Build history of the part. All positions in model axes, mm. A direction names the side the tool comes from. Give positions to 0.01 mm unless a question says otherwise; leave off trailing zeros. Order: outer loops, then holes, each group sorted by start corner. A loop starts at its lowest first (then second) coordinate and runs counter-clockwise, first axis right, second up. Notation, with made-up numbers: M 33,70 L 82,70 A30 ccw 82,98 Z; hole C 37,39.5 d1. An arc over 180 degrees is marked long. One line per item, written item: value.
from build123d import *

# Parameters (mm, degrees)
SKETCH2_R                = 37.75
SKETCH2_R_2              = 7.75
BOSS_EXTRUDE1_DEPTH      = 30
SKETCH3_R                = 1
CUT_EXTRUDE1_DEPTH       = 10
SKETCH4_R                = 1.5
BOSS_EXTRUDE2_DEPTH      = 5
FILLET1_R                = 10
CIRPATTERN1_COUNT        = 4
FILLET1_OF_CIRPATTERN1_R = 10


with BuildPart() as part:
    # Sketch2 → Boss-Extrude1 (new body)
    with BuildSketch(Plane.XY):
        Circle(SKETCH2_R)
        Circle(SKETCH2_R_2, mode=Mode.SUBTRACT)
    extrude(amount=BOSS_EXTRUDE1_DEPTH)

    # Sketch3 → Cut-Extrude1 (cut)
    with BuildSketch(Plane.XY.offset(30)):
        with Locations((0, 12.5)):
            Circle(SKETCH3_R)
        with Locations((10.825317547, -6.25)):
            Circle(SKETCH3_R)
        with Locations((-10.825317547, -6.25)):
            Circle(SKETCH3_R)
    extrude(amount=-CUT_EXTRUDE1_DEPTH, mode=Mode.SUBTRACT)

    # Sketch4 → Boss-Extrude2 (add)
    with BuildSketch(Plane(origin=(0, 0, 0), x_dir=(-1, 0, 0), z_dir=(0, 0, -1))):
        with BuildLine():
            Line((-4, 37.495028442), (0, 37.75))
            Line((0, 37.75), (4, 37.495028442))
            Line((4, 37.495028442), (4, 40))
            ThreePointArc((4, 40), (0, 44), (-4, 40))
            Line((-4, 40), (-4, 37.495028442))
        make_face()
        with Locations((0, 40)):
            Circle(SKETCH4_R, mode=Mode.SUBTRACT)
    boss_extrude2 = extrude(amount=-BOSS_EXTRUDE2_DEPTH)

    # Fillet1
    # the kernel refuses this fillet: 10 mm, written as the material it adds along each edge
    with BuildSketch(Plane(origin=(4, 37.537481269, 5), x_dir=(0.9825908408243521, -0.18578277511139904, 0), z_dir=(0, 0, -1))) as fillet1_piece_1:
        with BuildLine():
            CenterArc((6.893121156, -9.967448048), FILLET1_R, 94.624278966, 49.061773925)
            Line((-1.164720332, -4.045354621), (-1.970504481, -3.453145278))
            ThreePointArc((-1.970504481, -3.453145278), (-1.440084404, -2.233865576), (-0.982590841, 0.185782775))
            Line((-0.982590841, 0.185782775), (0.0806213, 0.996744805))
            ThreePointArc((0.0806213, 0.996744805), (3.043454077, 0.877116383), (6.006286855, 0.996744805))
            Line((6.006286855, 0.996744805), (6.086908155, 0))
        make_face()
    extrude(amount=5)
    with BuildSketch(Plane(origin=(-4, 37.537481269, 5), x_dir=(-0.9825908408243521, -0.185782775111399, 0), z_dir=(0, 0, -1))) as fillet1_piece_2:
        with BuildLine():
            CenterArc((6.893121156, 9.967448048), FILLET1_R, 216.31394711, 49.061773925)
            Line((-1.164720332, 4.045354621), (-1.970504481, 3.453145278))
            ThreePointArc((-1.970504481, 3.453145278), (-1.440084404, 2.233865576), (-0.982590841, -0.185782775))
            Line((-0.982590841, -0.185782775), (0.0806213, -0.996744805))
            ThreePointArc((0.0806213, -0.996744805), (3.043454077, -0.877116383), (6.006286855, -0.996744805))
            Line((6.006286855, -0.996744805), (6.086908155, 0))
        make_face()
    extrude(amount=5)

    # CirPattern1: Boss-Extrude2 ×4 about axis
    cirpattern1_axis = Axis((0, 0, 0), (0, 0, 1))
    for i in range(1, CIRPATTERN1_COUNT):
        add(boss_extrude2.rotate(cirpattern1_axis, i * 360 / CIRPATTERN1_COUNT))

    # Fillet1 of CirPattern1
    # the kernel refuses this fillet: 10 mm, written as the material it adds along each edge
    with BuildSketch(Plane(origin=(-37.537481269, 4, 5), x_dir=(0.18578277511140276, 0.9825908408243514, 0), z_dir=(0, 0, -1)), Plane(origin=(-4, -37.537481269, 5), x_dir=(-0.9825908408243512, 0.18578277511140392, 0), z_dir=(0, 0, -1)), Plane(origin=(37.537481269, -4, 5), x_dir=(-0.1857827751114012, -0.9825908408243518, 0), z_dir=(0, 0, -1))) as fillet1_of_cirpattern1_piece_1:
        with BuildLine():
            CenterArc((6.893121156, -9.967448048), FILLET1_OF_CIRPATTERN1_R, 94.624278966, 49.061773925)
            Line((-1.164720332, -4.045354621), (-1.970504481, -3.453145278))
            ThreePointArc((-1.970504481, -3.453145278), (-1.440084404, -2.233865576), (-0.982590841, 0.185782775))
            Line((-0.982590841, 0.185782775), (0.0806213, 0.996744805))
            ThreePointArc((0.0806213, 0.996744805), (3.043454077, 0.877116383), (6.006286855, 0.996744805))
            Line((6.006286855, 0.996744805), (6.086908155, 0))
        make_face()
    extrude(amount=5)
    with BuildSketch(Plane(origin=(-37.537481269, -4, 5), x_dir=(0.1857827751113977, -0.9825908408243523, 0), z_dir=(0, 0, -1)), Plane(origin=(4, -37.537481269, 5), x_dir=(0.9825908408243529, 0.18578277511139504, 0), z_dir=(0, 0, -1)), Plane(origin=(37.537481269, 4, 5), x_dir=(-0.18578277511139632, 0.9825908408243527, 0), z_dir=(0, 0, -1))) as fillet1_of_cirpattern1_piece_2:
        with BuildLine():
            CenterArc((6.893121156, 9.967448048), FILLET1_OF_CIRPATTERN1_R, 216.31394711, 49.061773925)
            Line((-1.164720332, 4.045354621), (-1.970504481, 3.453145278))
            ThreePointArc((-1.970504481, 3.453145278), (-1.440084404, 2.233865576), (-0.982590841, -0.185782775))
            Line((-0.982590841, -0.185782775), (0.0806213, -0.996744805))
            ThreePointArc((0.0806213, -0.996744805), (3.043454077, -0.877116383), (6.006286855, -0.996744805))
            Line((6.006286855, -0.996744805), (6.086908155, 0))
        make_face()
    extrude(amount=5)


solid = part.part
1) Saw through at A-A, the plane z = 3.5. Write the cut outline in (x, y), then the cut area to 3 significant figures.
Check values:
outline: M -41.73,-3.61 A10 cw -36.41,-9.98 A37.75 ccw -9.98,-36.41 A10 cw -3.61,-41.73 A4 ccw 3.61,-41.73 A10 cw 9.98,-36.41 A37.75 ccw 36.41,-9.98 A10 cw 41.73,-3.61 A4 ccw 41.73,3.61 A10 cw 36.41,9.98 A37.75 ccw 9.98,36.41 A10 cw 3.61,41.73 A4 ccw -3.61,41.73 A10 cw -9.98,36.41 A37.75 ccw -36.41,9.98 A10 cw -41.73,3.61 A4 ccw Z; hole C -40,0 d3; hole C 0,0 d15.5; hole C 0,-40 d3; hole C 0,40 d3; hole C 40,0 d3
area: 4,480 mm^2
2) Saw through at B-B, the plane y = 0. Write the cut outline in (x, z).
Check values:
outline: M -44,0 L -41.5,0 L -41.5,5 L -44,5 Z; M -38.5,0 L -7.75,0 L -7.75,30 L -37.75,30 L -37.75,5 L -38.5,5 Z; M 7.75,0 L 38.5,0 L 38.5,5 L 37.75,5 L 37.75,30 L 7.75,30 Z; M 41.5,0 L 44,0 L 44,5 L 41.5,5 Z
3) Drill centre lines: probe 1 along Y at (x, z) = (0, 3.05); probe 2 along Y at (x, z) = (10, 26.5); probe 3 along Y at (x, z) = (0, 19). Where is each one in solid material? Low to high. Write a range as from..to.
Check values:
probe 1: -44..-41.5, -38.5..-7.75, 7.75..38.5, 41.5..44
probe 2: -36.4..-6.81, -5.69..36.4
probe 3: -37.75..-7.75, 7.75..37.75
4) Saw through at D-D, the plane z = 24. Write the cut outline in (x, y), then the cut area to 3 significant figures.
Check values:
outline: C 0,0 d75.5; hole C -10.83,-6.25 d2; hole C 0,0 d15.5; hole C 0,12.5 d2; hole C 10.83,-6.25 d2
area: 4,280 mm^2
5) Tool access for faces 1 (the face through (6.17, -38.413, 2.535)), 2 (the face through (11, -6, 20)): list every direction of +Z, -Z, +X, -X, +Y, -Y with a clear straight run to the whole face (end or side of a thin tool).
Check values:
face 1: +Z, -Z, +X, -Y
face 2: +Z
6) Saw through at C-C, the plane x = 5. Write the cut outline in (y, z), then the cut area to 3 significant figures.
Check values:
outline: M -39.58,0 L -5.92,0 L -5.92,30 L -37.42,30 L -37.42,5 L -39.58,5 Z; M 5.92,0 L 39.58,0 L 39.58,5 L 37.42,5 L 37.42,30 L 5.92,30 Z
area: 1,910 mm^2
7) Pin check, flat tips, straight feed: pin 1 (4 mm diameter, centred on x = -40, y = -3.5, fed in from +Z); pin 2 (2 mm diameter, centred on y = -30, z = 18, fed in from +X); pin 3 (5 mm diameter, centred on x = 11, z = 9, fed in from -Y). Stop position of each tip, or through.
Check values:
pin 1: z = 5
pin 2: x = 24.17
pin 3: y = -36.78
8) Mould opens along Y. For faces 3 (the face through (0, -44, 2)), 4 (the face through (-1.009, 7.684, 14.79)), 5 (the face through (36.007, 11.339, 14.79)), 6 (the face through (38.413, 6.17, 2.535)) say: released by +Y, released by -Y, zero draft, split by the parting line, or undercut.
Check values:
face 3: released by -Y
face 4: undercut
face 5: split by the parting line
face 6: released by +Y
